from build123d import *

# Parameters (mm, degrees)
F0_R     = 1.6
F1_DEPTH = 3.175


with BuildPart() as f1:
    # F0 (on Top) → F1 (new body)
    with BuildSketch(Plane.XY):
        with BuildLine():
            Line((5, 7.5), (5, 13))
            ThreePointArc((5, 13), (3.397058, 16.275063), (0, 17.6))
            ThreePointArc((0, 17.6), (-3.397058, 16.275063), (-5, 13))
            Line((-5, 13), (-5, 7.5))
            ThreePointArc((-5, 7.5), (-5.732233, 5.732233), (-7.5, 5))
            Line((-7.5, 5), (-13, 5))
            ThreePointArc((-13, 5), (-16.275063, 3.397058), (-17.6, 0))
            ThreePointArc((-17.6, 0), (-16.275063, -3.397058), (-13, -5))
            Line((-13, -5), (-7.5, -5))
            ThreePointArc((-7.5, -5), (-5.732233, -5.732233), (-5, -7.5))
            Line((-5, -7.5), (-5, -13))
            ThreePointArc((-5, -13), (-3.397058, -16.275063), (0, -17.6))
            ThreePointArc((0, -17.6), (3.397058, -16.275063), (5, -13))
            Line((5, -13), (5, -7.5))
            ThreePointArc((5, -7.5), (5.732233, -5.732233), (7.5, -5))
            Line((7.5, -5), (13, -5))
            ThreePointArc((13, -5), (16.275063, -3.397058), (17.6, 0))
            ThreePointArc((17.6, 0), (16.275063, 3.397058), (13, 5))
            Line((13, 5), (7.5, 5))
            ThreePointArc((7.5, 5), (5.732233, 5.732233), (5, 7.5))
        make_face()
        with Locations((0, -13)):
            Circle(F0_R, mode=Mode.SUBTRACT)
        with Locations((0, -8)):
            Circle(F0_R, mode=Mode.SUBTRACT)
        with Locations((-13, 0)):
            Circle(F0_R, mode=Mode.SUBTRACT)
        with Locations((-8, 0)):
            Circle(F0_R, mode=Mode.SUBTRACT)
        Polygon((-2.313127, 1.150841), (-2.481189, 1.651718), (-1.954254, 1.689937), (-1.992473, 2.216873), (-1.472587, 2.122848), (-1.378562, 2.642733), (-0.898392, 2.422372), (-0.678031, 2.902541), (-0.267748, 2.56969), (0.065104, 2.979972), (0.37972, 2.555544), (0.804147, 2.87016), (1.003328, 2.380825), (1.492663, 2.580005), (1.563894, 2.056509), (2.08739, 2.12774), (2.026194, 1.602976), (2.550958, 1.54178), (2.361181, 1.048721), (2.85424, 0.858945), (2.547807, 0.428572), (2.97818, 0.122139), (2.574344, -0.218506), (2.914989, -0.622342), (2.439126, -0.851855), (2.668639, -1.327718), (2.150649, -1.431678), (2.254609, -1.949669), (1.727038, -1.921544), (1.698914, -2.449115), (1.194912, -2.290672), (1.036469, -2.794674), (0.587704, -2.515869), (0.308899, -2.964634), (-0.056431, -2.582985), (-0.43808, -2.948314), (-0.69702, -2.487802), (-1.157533, -2.746742), (-1.293813, -2.236301), (-1.804254, -2.372581), (-1.809311, -1.844285), (-2.337607, -1.849342), (-2.211123, -1.336386), (-2.724079, -1.209903), (-2.474002, -0.744517), (-2.939388, -0.494441), (-2.581431, -0.105868), (-2.970004, 0.252089), (-2.526659, 0.539434), (-2.814004, 0.982779), align=None, mode=Mode.SUBTRACT)
        with Locations((8, 0)):
            Circle(F0_R, mode=Mode.SUBTRACT)
        with Locations((0, 8)):
            Circle(F0_R, mode=Mode.SUBTRACT)
        with Locations((13, 0)):
            Circle(F0_R, mode=Mode.SUBTRACT)
        with Locations((0, 13)):
            Circle(F0_R, mode=Mode.SUBTRACT)
    extrude(amount=F1_DEPTH)


solid = f1.part
Design review of the part built by this model. Coordinates are the model's own, in mm. A direction names the side the tool comes from. Coordinates: 2 decimals unless noted, no trailing zeros. Write each loop counter-clockwise with the first axis right and the second up, starting at its lowest first coordinate (ties: lowest second). Pieces come first, ordered by that corner, then holes. Notation, with made-up numbers: (-2.5, 49) - (18.5, 49) arc R20 ccw to (18.5, 66) - close; hole circle Ø2 at (66.5, -9). An arc over 180 degrees is marked (long way). One line per item, written item: value.
1) Mouldability with a two-part tool opening along Y and no side actions: class faces 1 (the face through (5.713, -5.752, 1.565)), 2 (the face through (-9.6, 0.07, 1.57)), 3 (the face through (-0.35, -14.56, 1.57)), 4 (the face through (0, -4, 0)) as +Y half, -Y half, draft (parallel to the pull), parting line (faces both ways), or undercut.
Answer sheet:
face 1: -Y half
face 2: undercut
face 3: undercut
face 4: draft
2) To check wall thickness, follow probe 1 along Y at (x, z) = (-13, 2.45); probe 2 along X at (y, z) = (14, 3.05); probe 3 along X at (y, z) = (9, 0.4). State the ranges of each line that lie inside material, in increasing order.
Answer sheet:
probe 1: y = -5 to -1.6, 1.6 to 5
probe 2: x = -4.81 to -1.25, 1.25 to 4.81
probe 3: x = -5 to -1.25, 1.25 to 5
3) Add section A-A (y = 8). State the section outline as (x, z) points (3 decimals).
Answer sheet:
outline: (-5, 0) - (-1.6, 0) - (-1.6, 3.175) - (-5, 3.175) - close; (1.6, 0) - (5, 0) - (5, 3.175) - (1.6, 3.175) - close
4) Insertion check: pin 1 (1.5 mm diameter, centred on x = 7.5, y = -7.5, fed in from -Z); pin 2 (1.6 mm diameter, centred on x = -10.5, z = 1.5, fed in from -Y); pin 3 (1.6 mm diameter, centred on x = -11, z = 1, fed in from +Y). Each pin has a flat end and moves straight along its axis. Give the tip position at first contact, or say it passes through.
Answer sheet:
pin 1: passes through
pin 2: stops at y = -5
pin 3: stops at y = 5
5) Add section D-D (y = -4.5). State the section outline as (x, z) points (3 decimals), plus the area to 3 significant figures.
Answer sheet:
outline: (-14.802, 0) - (14.802, 0) - (14.802, 3.175) - (-14.802, 3.175) - close
area: 94.0 mm2
6) Add section C-C (z = 1.4). Give the number of separate pieces and of enclosed holes in the cut face, plus the area to 3 significant figures.
Answer sheet:
separate pieces: 1
enclosed holes: 9
area: 478 mm2
7) For faces 5 (the face through (-5, -10, 2)), 6 (the face through (10, -5, 2)), 7 (the face through (-5, 10, 2)), 8 (the face through (10, 5, 2)), list the 3-axis set-ups (+Z, -Z, +X, -X, +Y, -Y) from which the entire face can be reached by the end or side of a thin tool; tool diameter is ignored.
Answer sheet:
face 5: +Z, -Z, -X, -Y
face 6: +Z, -Z, +X, -Y
face 7: +Z, -Z, -X, +Y
face 8: +Z, -Z, +X, +Y
